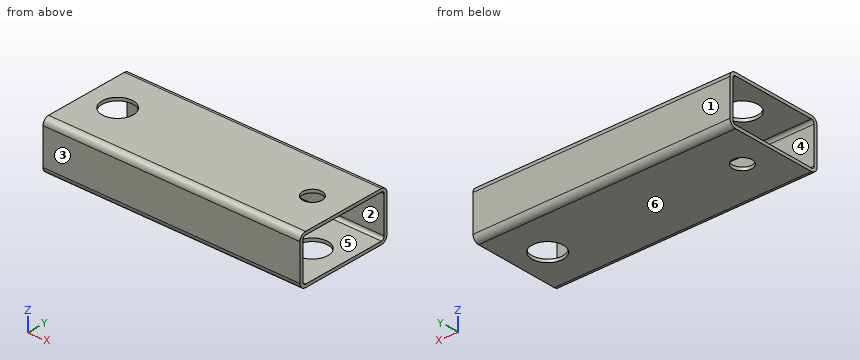
from build123d import *

# Parameters (mm, degrees)
RECTANGULAR_TUBE_2_50_X_25_X_1_6_1_DEPTH = 132
SKETCH2_R                                = 5
CUT_EXTRUDE1_DEPTH                       = 137.65284483
SKETCH2_3_R                              = 8
SKETCH2_3_R_2                            = 5
CUT_EXTRUDE2_DEPTH                       = 1.6
CUT_EXTRUDE5_START                       = -23.4
SKETCH2_4_R                              = 8
SKETCH2_4_R_2                            = 5
CUT_EXTRUDE5_DEPTH                       = 1.6


with BuildPart() as part:
    # Sketch14 → Rectangular tube 2 50 X 25 X 1.6(1) (new body)
    with BuildSketch(Plane(origin=(0, 0, 0), x_dir=(0, 0, -1), z_dir=(1, 0, 0))):
        with BuildLine():
            Line((-9.3, -25), (9.3, -25))
            ThreePointArc((9.3, -25), (11.5627417, -24.0627417), (12.5, -21.8))
            Line((12.5, -21.8), (12.5, 21.8))
            ThreePointArc((12.5, 21.8), (11.5627417, 24.0627417), (9.3, 25))
            Line((9.3, 25), (-9.3, 25))
            ThreePointArc((-9.3, 25), (-11.5627417, 24.0627417), (-12.5, 21.8))
            Line((-12.5, 21.8), (-12.5, -21.8))
            ThreePointArc((-12.5, -21.8), (-11.5627417, -24.0627417), (-9.3, -25))
        make_face()
        with BuildLine():
            Line((-9.3, -23.4), (9.3, -23.4))
            ThreePointArc((9.3, -23.4), (10.43137085, -22.93137085), (10.9, -21.8))
            Line((10.9, -21.8), (10.9, 21.8))
            ThreePointArc((10.9, 21.8), (10.43137085, 22.93137085), (9.3, 23.4))
            Line((9.3, 23.4), (-9.3, 23.4))
            ThreePointArc((-9.3, 23.4), (-10.43137085, 22.93137085), (-10.9, 21.8))
            Line((-10.9, 21.8), (-10.9, -21.8))
            ThreePointArc((-10.9, -21.8), (-10.43137085, -22.93137085), (-9.3, -23.4))
        make_face(mode=Mode.SUBTRACT)
    extrude(amount=RECTANGULAR_TUBE_2_50_X_25_X_1_6_1_DEPTH)

    # Sketch2 → Cut-Extrude1 (cut, through all)
    with BuildSketch(Plane.XY.offset(12.5)):
        with Locations((16, 0)):
            Circle(SKETCH2_R)
        with Locations((116, 0)):
            Circle(SKETCH2_R)
    extrude(amount=-CUT_EXTRUDE1_DEPTH, mode=Mode.SUBTRACT)

    # Sketch2<3> → Cut-Extrude2 (cut)
    # profile 1 of 2: a face of its own
    with BuildSketch(Plane.XY.offset(12.5)):
        with Locations((16, 0)):
            Circle(SKETCH2_3_R)
        with Locations((16, 0)):
            Circle(SKETCH2_3_R_2, mode=Mode.SUBTRACT)
    # profile 2 of 2: a face of its own
    with BuildSketch(Plane.XY.offset(12.5)):
        with Locations((16, 0)):
            Circle(SKETCH2_3_R_2)
    extrude(amount=-CUT_EXTRUDE2_DEPTH, mode=Mode.SUBTRACT)

    # Sketch2<4> → Cut-Extrude5 (cut)
    # profile 1 of 2: a face of its own
    with BuildSketch(Plane.XY.offset(12.5).offset(CUT_EXTRUDE5_START)):
        with Locations((116, 0)):
            Circle(SKETCH2_4_R)
        with Locations((116, 0)):
            Circle(SKETCH2_4_R_2, mode=Mode.SUBTRACT)
    # profile 2 of 2: a face of its own
    with BuildSketch(Plane.XY.offset(12.5).offset(CUT_EXTRUDE5_START)):
        with Locations((116, 0)):
            Circle(SKETCH2_4_R_2)
    extrude(amount=-CUT_EXTRUDE5_DEPTH, mode=Mode.SUBTRACT)


solid = part.part
Part model, mm, in its own coordinate system. Face numbers are marked on the shaded views. A direction names the side the tool comes from. Give positions to 0.01 mm unless a question says otherwise; leave off trailing zeros. Order: outer loops, then holes, each group sorted by start corner. A loop starts at its lowest first (then second) coordinate and runs counter-clockwise, first axis right, second up. Notation, with made-up numbers: (-25.75, -1) - (-20.75, -1) arc R19 cw to (-20.75, 15) - close; hole circle Ø2 at (77, 17.5). An arc over 180 degrees is marked (long way). Use a Markdown table: item, result.
1) Flat gauge pins, fed straight in: P1, Ø11.5, axis at x = 16, y = 0, coming from the +Z side; P2, Ø14.5, axis at x = 116, y = 0, coming from the -Z side; P3, Ø9, axis at x = 116, y = 0, coming from the -Z side. Where does each tip first touch, or does it go through?
Checked values:
| item | result |
|---|---|
| P1 | z = -10.9 |
| P2 | z = 10.9 |
| P3 | through |
2) Saw through at C-C on z = -4. List the corners of the cut face in (x, y).
Checked values:
| item | result |
|---|---|
| outline | (0, -25) - (132, -25) - (132, -23.4) - (0, -23.4) - close; (0, 23.4) - (132, 23.4) - (132, 25) - (0, 25) - close |
3) Saw through at A-A on y = 0. List the corners of the cut face in (x, z).
Checked values:
| item | result |
|---|---|
| outline | (0, -12.5) - (11, -12.5) - (11, -10.9) - (0, -10.9) - close; (0, 10.9) - (8, 10.9) - (8, 12.5) - (0, 12.5) - close; (21, -12.5) - (108, -12.5) - (108, -10.9) - (21, -10.9) - close; (24, 10.9) - (111, 10.9) - (111, 12.5) - (24, 12.5) - close; (121, 10.9) - (132, 10.9) - (132, 12.5) - (121, 12.5) - close; (124, -12.5) - (132, -12.5) - (132, -10.9) - (124, -10.9) - close |
4) Probe L1, parallel to Y at x = 23.5, z = -8.25; L2, parallel to Z at x = 75.5, y = 3.5; L3, parallel to Z at x = 14, y = 7. List the from-to ranges inside material, lowest first. Write a range as from..to.
Checked values:
| item | result |
|---|---|
| L1 | -25..-23.4, 23.4..25 |
| L2 | -12.5..-10.9, 10.9..12.5 |
| L3 | -12.5..-10.9 |
5) Saw through at D-D on y = -18. List the corners of the cut face in (x, z), plus the area to 3 significant figures.
Checked values:
| item | result |
|---|---|
| outline | (0, -12.5) - (132, -12.5) - (132, -10.9) - (0, -10.9) - close; (0, 10.9) - (132, 10.9) - (132, 12.5) - (0, 12.5) - close |
| area | 422 mm² |
6) Two-plate mould, pull along Y, no slides. Class the marked faces 3, 4, 5 and 6: +Y half, -Y half, draft (parallel to the pull), parting line (faces both ways), or undercut.
Checked values:
| item | result |
|---|---|
| face 3 | -Y half |
| face 4 | undercut |
| face 5 | undercut |
| face 6 | draft |
7) Saw through at B-B on x = 116. List the corners of the cut face in (y, z).
Checked values:
| item | result |
|---|---|
| outline | (-25, -9.3) arc R3.2 ccw to (-21.8, -12.5) - (-8, -12.5) - (-8, -10.9) - (-21.8, -10.9) arc R1.6 cw to (-23.4, -9.3) - (-23.4, 9.3) arc R1.6 cw to (-21.8, 10.9) - (-5, 10.9) - (-5, 12.5) - (-21.8, 12.5) arc R3.2 ccw to (-25, 9.3) - close; (5, 10.9) - (21.8, 10.9) arc R1.6 cw to (23.4, 9.3) - (23.4, -9.3) arc R1.6 cw to (21.8, -10.9) - (8, -10.9) - (8, -12.5) - (21.8, -12.5) arc R3.2 ccw to (25, -9.3) - (25, 9.3) arc R3.2 ccw to (21.8, 12.5) - (5, 12.5) - close |
8) 3-axis set-ups, long thin cutter, end or side, ignore diameter. For the marked faces 1 and 2: which of +Z, -Z, +X, -X, +Y, -Y reach the whole face in a straight line?
Checked values:
| item | result |
|---|---|
| face 1 | +Z, -Z, +X, -X, +Y |
| face 2 | +X, -X |
